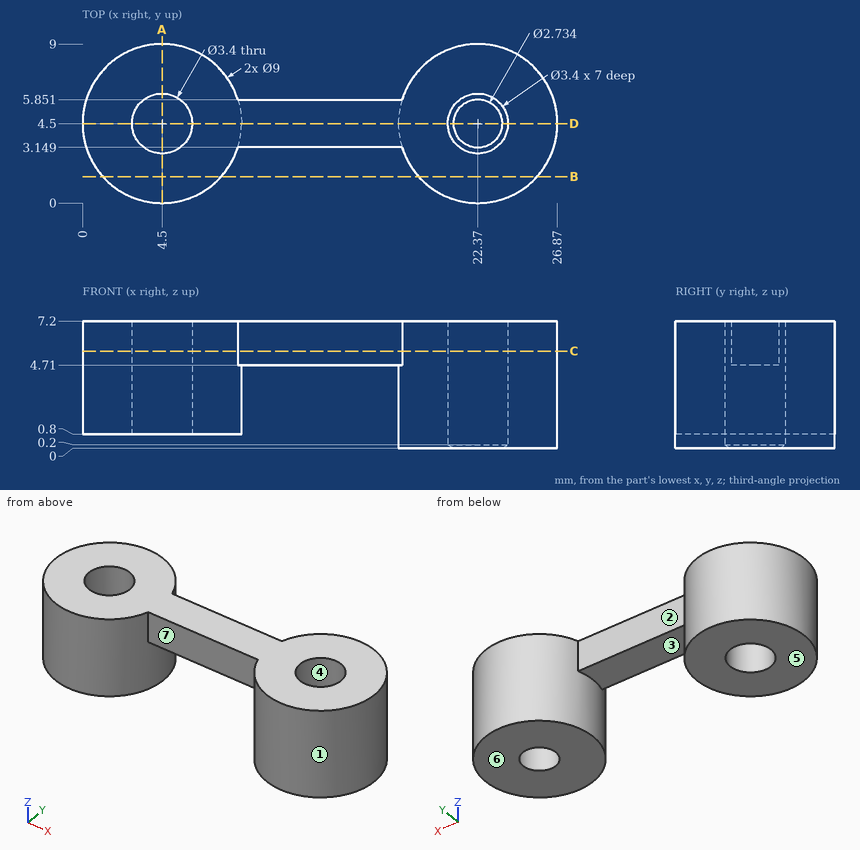
Verification items for this drawing (mm, ordinates from the low corner). A direction names the side the tool comes from. Coordinates: 2 decimals unless noted, no trailing zeros. Order: outer loops, then holes, each group sorted by start corner. A loop starts at its lowest first (then second) coordinate and runs counter-clockwise, first axis right, second up. Notation, with made-up numbers: (77, -17.75) -> (118, -17.75) arc R21 ccw to (118, -9.75) -> close; hole circle Ø2 at (82, -26.5). An arc over 180 degrees is marked (long way). Answer as CSV lines item,"result". Start each with the question number.
1) Set-up check for the marked faces 5, 6 and 7: record each of +Z, -Z, +X, -X, +Y, -Y from which the full face is reachable in a straight line by a thin tool's end or side.
2) Release check for a two-part mould opening along Y. For the marked faces 1, 2, 3 and 4 record: released by +Y, released by -Y, zero draft, split by the parting line, or undercut.
3) Gauge pin test, flat ends, axial feed: pin 1 Ø3 at (x, y) = (14, 5) entering from -Z; pin 2 Ø1 at (x, z) = (14, 6) entering from -Y; pin 3 Ø2 at (x, z) = (13, 5.5) entering from +Y; pin 4 Ø4.5 at (x, y) = (22.37, 4.5) entering from +Z. Record the tip position at first contact, or that the pin passes through.
4) Cross-section at A-A, the plane x = 4.5. Record the boundary of the cut face in (y, z).
5) Cross-section at B-B, the plane y = 1.5. Record the boundary of the cut face in (x, z).
6) Cross-section at C-C, the plane z = 5.5. Record the boundary of the cut face in (x, y).
7) Material ranges on L1, parallel to X at y = 4.5, z = 3; L2, parallel to X at y = 4.5, z = 5.5; L3, parallel to Y at x = 4.5, z = 4.75, recorded low to high. Write a range as [from, to].
8) Cross-section at D-D, the plane y = 4.5. Record the boundary of the cut face in (x, z).
Conclusion:
1,face 5,"-Z, -X, +Y, -Y"
1,face 6,"-Z, +X, -X, +Y, -Y"
1,face 7,"+Z, -Z, -Y"
2,face 1,"split by the parting line"
2,face 2,"released by +Y"
2,face 3,"zero draft"
2,face 4,"undercut"
3,pin 1,"stops at z = 4.71"
3,pin 2,"stops at y = 3.15"
3,pin 3,"stops at y = 5.85"
3,pin 4,"stops at z = 7.2"
4,outline,"(0, 0.8) -> (2.8, 0.8) -> (2.8, 7.2) -> (0, 7.2) -> close; (6.2, 0.8) -> (9, 0.8) -> (9, 7.2) -> (6.2, 7.2) -> close"
5,outline,"(1.15, 0.8) -> (7.85, 0.8) -> (7.85, 7.2) -> (1.15, 7.2) -> close; (19.02, 0) -> (25.72, 0) -> (25.72, 7.2) -> (19.02, 7.2) -> close"
6,outline,"(8.79, 3.15) -> (18.08, 3.15) arc R4.5 ccw (long way) to (18.08, 5.85) -> (8.79, 5.85) arc R4.5 ccw (long way) to start; hole circle Ø3.4 at (4.5, 4.5); hole circle Ø3.4 at (22.37, 4.5)"
7,L1,"x = [0, 2.8], [6.2, 9], [17.87, 20.67], [24.07, 26.87]"
7,L2,"x = [0, 2.8], [6.2, 20.67], [24.07, 26.87]"
7,L3,"y = [0, 2.8], [6.2, 9]"
8,outline,"(0, 0.8) -> (2.8, 0.8) -> (2.8, 7.2) -> (0, 7.2) -> close; (6.2, 0.8) -> (9, 0.8) -> (9, 4.71) -> (17.87, 4.71) -> (17.87, 0) -> (21, 0) -> (20.67, 0.2) -> (20.67, 7.2) -> (6.2, 7.2) -> close; (23.74, 0) -> (26.87, 0) -> (26.87, 7.2) -> (24.07, 7.2) -> (24.07, 0.2) -> close"
